Read the model definition and answer for the solid it produces. Units are mm, in the model's axes. Coordinates: 2 decimals unless noted, no trailing zeros. Write each loop counter-clockwise with the first axis right and the second up, starting at its lowest first coordinate (ties: lowest second). Pieces come first, ordered by that corner, then holes. Notation, with made-up numbers: (15, 3) - (46, 3) arc R18 cw to (46, 30) - close; hole circle Ø9 at (67, -5). An arc over 180 degrees is marked (long way). Use a Markdown table: item, result.
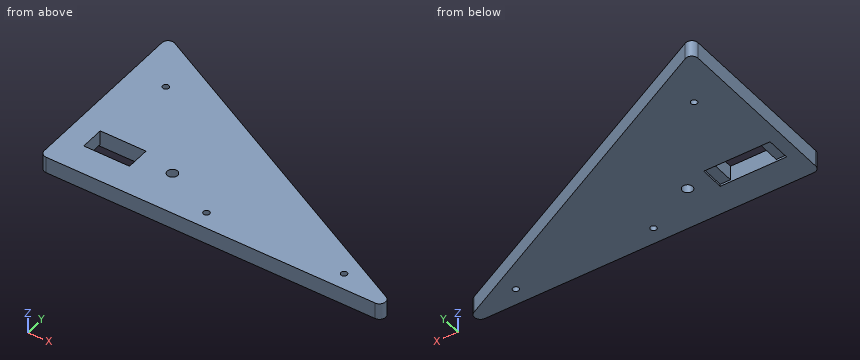
from build123d import *

# Parameters (mm, degrees)
BOSS_EXTRUDE1_DEPTH     = 8
CUT_EXTRUDE6_DEPTH      = 30
CUT_EXTRUDE6_DEPTH_BACK = 30
SKETCH3_R               = 1.5
SKETCH8_R               = 2.25
CUT_EXTRUDE9_DEPTH      = 20
SKETCH11_W              = 5
SKETCH11_H              = 11.5
CUT_EXTRUDE10_DEPTH     = 1
SKETCH8_6_R             = 1.5
CUT_EXTRUDE11_DEPTH     = 10
SKETCH12_R              = 2.5
CUT_EXTRUDE12_DEPTH     = 20


with BuildPart() as part:
    # Sketch1 → Boss-Extrude1 (new body)
    with BuildSketch(Plane.XY):
        with BuildLine():
            Line((-67.152143845, 0), (92.454966604, 0))
            ThreePointArc((92.454966604, 0), (95.370750394, 2.294163695), (93.827010641, 5.667863407))
            Line((93.827010641, 5.667863407), (-65.780099807, 87.751520209))
            ThreePointArc((-65.780099807, 87.751520209), (-68.714812698, 87.64452893), (-70.152143845, 85.083656802))
            Line((-70.152143845, 85.083656802), (-70.152143845, 3))
            ThreePointArc((-70.152143845, 3), (-69.273464189, 0.878679656), (-67.152143845, 0))
        make_face()
    extrude(amount=BOSS_EXTRUDE1_DEPTH)

    # Sketch3 → Cut-Extrude6 (cut, two sides: drawn at the far end of the back side and taken through both)
    with BuildSketch(Plane.XY.offset(-CUT_EXTRUDE6_DEPTH_BACK)):
        with Locations(Location((71.800150685, 8, 0), (0, 0, 180))):
            Circle(SKETCH3_R)
        with Locations(Location((5.050150685, 8, 0), (0, 0, 180))):
            Circle(SKETCH3_R)
    extrude(amount=CUT_EXTRUDE6_DEPTH + CUT_EXTRUDE6_DEPTH_BACK, mode=Mode.SUBTRACT)

    # Sketch8 → Cut-Extrude9 (cut)
    # profile 1 of 5: a face of its own
    with BuildSketch(Plane.XY.offset(8)):
        with BuildLine():
            Line((-53.152143845, 14.324774739), (-36.702143845, 14.324774739))
            Line((-36.702143845, 14.324774739), (-36.702143845, 25.824774739))
            Line((-36.702143845, 25.824774739), (-53.152143845, 25.824774739))
            ThreePointArc((-53.152143845, 25.824774739), (-49.847541871, 24.780314644), (-47.743470295, 22.026376755))
            ThreePointArc((-47.743470295, 22.026376755), (-45.112924044, 20.074774739), (-47.743470295, 18.123172724))
            ThreePointArc((-47.743470295, 18.123172724), (-49.847541871, 15.369234835), (-53.152143845, 14.324774739))
        make_face()
    # profile 2 of 5: a face of its own
    with BuildSketch(Plane.XY.offset(8)):
        with BuildLine():
            ThreePointArc((-58.902143845, 20.074774739), (-57.218007837, 24.140638731), (-53.152143845, 25.824774739))
            Line((-53.152143845, 25.824774739), (-58.902143845, 25.824774739))
            Line((-58.902143845, 25.824774739), (-58.902143845, 20.074774739))
        make_face()
    # profile 3 of 5: a face of its own
    with BuildSketch(Plane.XY.offset(8)):
        with BuildLine():
            Line((-58.902143845, 14.324774739), (-53.152143845, 14.324774739))
            ThreePointArc((-53.152143845, 14.324774739), (-57.218007837, 16.008910748), (-58.902143845, 20.074774739))
            Line((-58.902143845, 20.074774739), (-58.902143845, 14.324774739))
        make_face()
    # profile 4 of 5: a face of its own
    with BuildSketch(Plane.XY.offset(8)):
        with BuildLine():
            ThreePointArc((-47.743470295, 18.123172724), (-45.112924044, 20.074774739), (-47.743470295, 22.026376755))
            ThreePointArc((-47.743470295, 22.026376755), (-58.902143845, 20.074774739), (-47.743470295, 18.123172724))
        make_face()
        with Locations((-53.152143845, 20.074774739)):
            Circle(SKETCH8_R, mode=Mode.SUBTRACT)
    # profile 5 of 5: a face of its own
    with BuildSketch(Plane.XY.offset(8)):
        with Locations((-53.152143845, 20.074774739)):
            Circle(SKETCH8_R)
    extrude(amount=-CUT_EXTRUDE9_DEPTH, mode=Mode.SUBTRACT)

    # Sketch11 → Cut-Extrude10 (cut)
    with BuildSketch(Plane(origin=(0, 0, 0), x_dir=(-1, 0, 0), z_dir=(0, 0, -1))):
        with Locations((61.402143845, 20.074774739)):
            Rectangle(SKETCH11_W, SKETCH11_H)
        with Locations((34.202143845, 20.074774739)):
            Rectangle(SKETCH11_W, SKETCH11_H)
    extrude(amount=-CUT_EXTRUDE10_DEPTH, mode=Mode.SUBTRACT)

    # Sketch8_6 → Cut-Extrude11 (cut)
    with BuildSketch(Plane.XY.offset(8)):
        with Locations((-53.152143845, 63.365389143)):
            Circle(SKETCH8_6_R)
    extrude(amount=-CUT_EXTRUDE11_DEPTH, mode=Mode.SUBTRACT)

    # Sketch12 → Cut-Extrude12 (cut)
    with BuildSketch(Plane.XY.offset(8)):
        with Locations((-20.152143845, 20.5)):
            Circle(SKETCH12_R)
    extrude(amount=-CUT_EXTRUDE12_DEPTH, mode=Mode.SUBTRACT)


solid = part.part
(1) A cutting plane is placed at C-C, the plane z = 3.5. Write down the section's boundary in (x, y).
Report:
| item | result |
|---|---|
| outline | (-70.15, 3) arc R3 ccw to (-67.15, 0) - (92.45, 0) arc R3 ccw to (93.83, 5.67) - (-65.78, 87.75) arc R3 ccw to (-70.15, 85.08) - close; hole (-58.9, 14.32) - (-36.7, 14.32) - (-36.7, 25.82) - (-58.9, 25.82) - close; hole circle Ø3 at (-53.15, 63.37); hole circle Ø5 at (-20.15, 20.5); hole circle Ø3 at (5.05, 8); hole circle Ø3 at (71.8, 8) |
(2) Each of these flat-tipped pins is pushed along its axis until it touches: P1, Ø6.5, axis at x = -20.15, y = 20.5, coming from the +Z side; P2, Ø4, axis at x = -60.5, y = 21.5, coming from the -Z side; P3, Ø1.1, axis at y = 21, z = 0.5, coming from the +X side; P4, Ø4, axis at x = -46, z = 3, coming from the +Y side. Where does it stop, or does it pass through?
Report:
| item | result |
|---|---|
| P1 | stops at z = 8 |
| P2 | stops at z = 1 |
| P3 | stops at x = 65.08 |
| P4 | stops at y = 78.61 |
(3) A cutting plane is placed at D-D, the plane x = 24. Write down the section's boundary in (y, z), and give its area (3 significant figures).
Report:
| item | result |
|---|---|
| outline | (0, 0) - (41.58, 0) - (41.58, 8) - (0, 8) - close |
| area | 333 mm² |
(4) Straight lines are drawn through the part: L1, parallel to Y at x = 71, z = 6.75; L2, parallel to Y at x = 16, z = 5; L3, parallel to X at y = 36, z = 4.5. For each, find the intervals that lie inside material, in ascending order.
Report:
| item | result |
|---|---|
| L1 | y = 0 to 6.73, 9.27 to 17.41 |
| L2 | y = 0 to 45.69 |
| L3 | x = -70.15 to 34.85 |
(5) A cutting plane is placed at B-B, the plane x = -19.5. Write down the section's boundary in (y, z), and give its area (3 significant figures).
Report:
| item | result |
|---|---|
| outline | (0, 0) - (18.09, 0) - (18.09, 8) - (0, 8) - close; (22.91, 0) - (63.95, 0) - (63.95, 8) - (22.91, 8) - close |
| area | 473 mm² |
(6) A cutting plane is placed at A-A, the plane y = 20.5. Write down the section's boundary in (x, z).
Report:
| item | result |
|---|---|
| outline | (-70.15, 0) - (-63.9, 0) - (-63.9, 1) - (-58.9, 1) - (-58.9, 8) - (-70.15, 8) - close; (-36.7, 1) - (-31.7, 1) - (-31.7, 0) - (-22.65, 0) - (-22.65, 8) - (-36.7, 8) - close; (-17.65, 0) - (64.99, 0) - (64.99, 8) - (-17.65, 8) - close |
